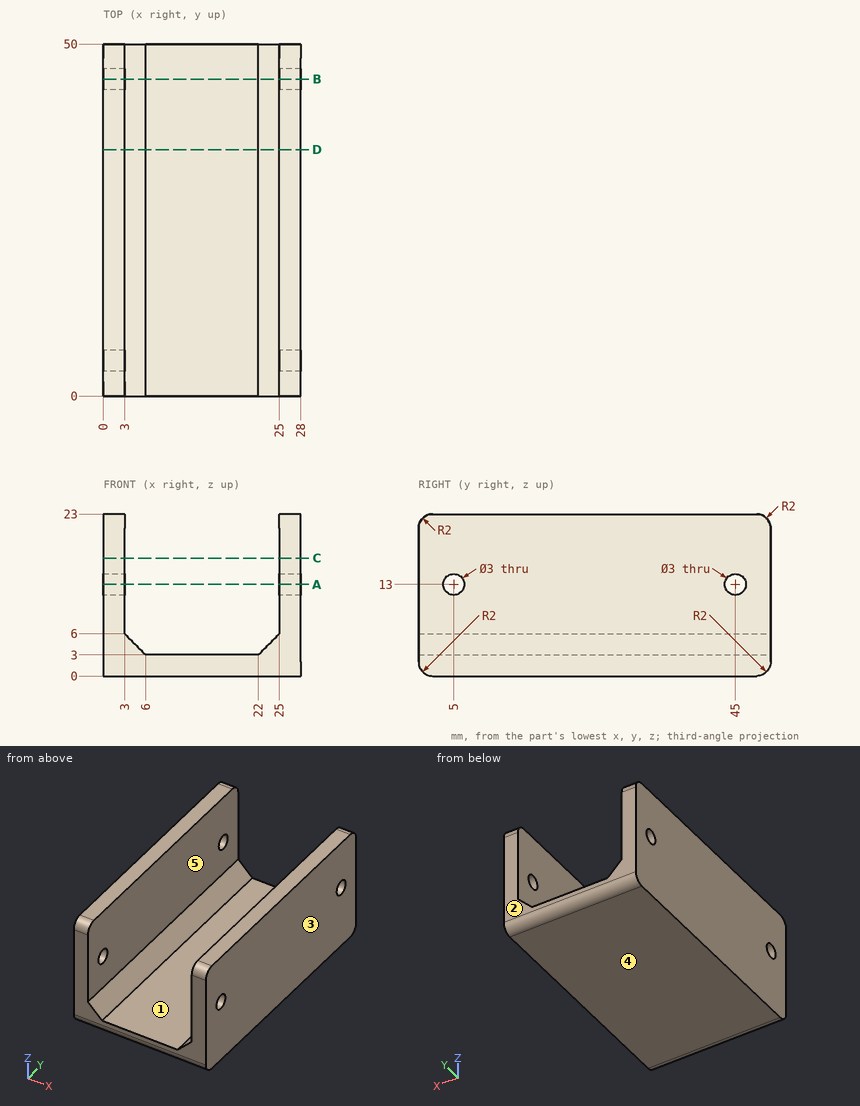
Check sheet for the drawn part. Datum: minimum x, y, z corner. Units: mm. A direction names the side the tool comes from. Coordinates: 2 decimals unless noted, no trailing zeros. Write each loop counter-clockwise with the first axis right and the second up, starting at its lowest first coordinate (ties: lowest second). Pieces come first, ordered by that corner, then holes. Notation, with made-up numbers: (77.5, 8.5) - (82.5, 8.5) arc R18 ccw to (82.5, 23.5) - close; hole circle Ø1 at (15, -27.5). An arc over 180 degrees is marked (long way). Answer as a JSON object with one key per item and string values.
(1) Cross-section at B-B on y = 45. Record the cut outline in (x, z), plus the area to 3 significant figures.
Report:
{"outline": "(0, 0) - (28, 0) - (28, 11.5) - (25, 11.5) - (25, 6) - (22, 3) - (6, 3) - (3, 6) - (3, 11.5) - (0, 11.5) - close; (0, 14.5) - (3, 14.5) - (3, 23) - (0, 23) - close; (25, 14.5) - (28, 14.5) - (28, 23) - (25, 23) - close", "area": "195 mm^2"}
(2) Tool access check on the marked faces 4 and 5. Record the directions out of +Z, -Z, +X, -X, +Y, -Y that give a thin tool (end or side, any length) a straight path to the whole face; none if there is none.
Report:
{"face 4": "-Z, +X, -X, +Y, -Y", "face 5": "+Z, +Y, -Y"}
(3) Cross-section at D-D on y = 35. Record the cut outline in (x, z).
Report:
{"outline": "(0, 0) - (28, 0) - (28, 23) - (25, 23) - (25, 6) - (22, 3) - (6, 3) - (3, 6) - (3, 23) - (0, 23) - close"}
(4) Cross-section at A-A on z = 13. Record the cut outline in (x, y), plus the area to 3 significant figures.
Report:
{"outline": "(0, 0) - (3, 0) - (3, 3.5) - (0, 3.5) - close; (0, 6.5) - (3, 6.5) - (3, 43.5) - (0, 43.5) - close; (0, 46.5) - (3, 46.5) - (3, 50) - (0, 50) - close; (25, 0) - (28, 0) - (28, 3.5) - (25, 3.5) - close; (25, 6.5) - (28, 6.5) - (28, 43.5) - (25, 43.5) - close; (25, 46.5) - (28, 46.5) - (28, 50) - (25, 50) - close", "area": "264 mm^2"}
(5) Mould release check, pull along X, two halves, no side actions. Record for the marked faces 1, 2 and 3: pulls with the +X half, pulls with the -X half, needs draft (parallel to the pull), parting line crosses it, or undercut.
Report:
{"face 1": "undercut", "face 2": "needs draft", "face 3": "pulls with the +X half"}
(6) Cross-section at C-C on z = 16.75. Record the cut outline in (x, y).
Report:
{"outline": "(0, 0) - (3, 0) - (3, 50) - (0, 50) - close; (25, 0) - (28, 0) - (28, 50) - (25, 50) - close"}
(7) Thickness scan on line 1 along Y through (x, z) = (25.8, 13); line 2 along X through (y, z) = (37.5, 12.5); line 3 along X through (y, z) = (16, 3.25). Record the ranges inside material, lowest first.
Report:
{"line 1": "0 to 3.5, 6.5 to 43.5, 46.5 to 50", "line 2": "0 to 3, 25 to 28", "line 3": "0 to 5.75, 22.25 to 28"}
(8) Gauge pin test, flat ends, axial feed: pin 1 Ø13 at (x, y) = (13.5, 18) entering from +Z; pin 2 Ø8 at (x, z) = (16, 9.5) entering from +Y. Record the tip position at first contact, or that the pin passes through.
Report:
{"pin 1": "z = 3", "pin 2": "through"}
